```python
from build123d import *

# Parameters (mm, degrees)
F0_W     = 17.78
F0_H     = 73.152
F0_H_2   = 5.08
F1_DEPTH = 5.08
F2_DEPTH = 10.16
F4_DEPTH = 25.4


# Not quite as in the source:
# - a feature names something its author has since deleted; it is built from what else it names


with BuildPart() as f1:
    # F0 (on Top) → F1 (new body)
    with BuildSketch(Plane.XY):
        with Locations((8.89, -41.656)):
            Rectangle(F0_W, F0_H)
        with Locations((8.89, -2.54)):
            Rectangle(F0_W, F0_H_2)
        with Locations((8.89, -114.808)):
            Rectangle(F0_W, F0_H)
        with Locations((8.89, -153.924)):
            Rectangle(F0_W, F0_H_2)
    extrude(amount=-F1_DEPTH)

    # F0 (on Top) → F2 (join)
    with BuildSketch(Plane.XY):
        with Locations((8.89, -2.54)):
            Rectangle(F0_W, F0_H_2)
        with Locations((8.89, -153.924)):
            Rectangle(F0_W, F0_H_2)
    extrude(amount=F2_DEPTH)

    # F3 (on face) → F4 (cut)
    with BuildSketch(Plane(origin=(0, 0, 0), x_dir=(0, -1, 0), z_dir=(-1, 0, 0))):
        Polygon((3.048, 9.144), (5.08, 2.54), (5.08, 9.144), align=None)
        Polygon((151.384, 9.144), (151.384, 2.54), (153.416, 9.144), align=None)
    extrude(amount=-F4_DEPTH, mode=Mode.SUBTRACT)


solid = f1.part
```
Geometry check sheet. Reference: the model listing, model coordinates, mm. A direction names the side the tool comes from. Coordinates: 2 decimals unless noted, no trailing zeros. Loops run counter-clockwise (first coordinate to the right, second up) from the corner with the lowest first, then second, coordinate; pieces in that order, holes last. Notation, with made-up numbers: (-27.75, 12.25) -> (28.25, 12.25) arc R14 ccw to (28.25, 19.25) -> close; hole circle Ø4 at (-36.75, 89.25). An arc over 180 degrees is marked (long way). Put each result on its own line as item: value.
1) Cross-section at C-C on y = -121.5. Record the boundary of the cut face in (x, z).
Result set:
outline: (0, -5.08) -> (17.78, -5.08) -> (17.78, 0) -> (0, 0) -> close
2) Release check for a two-part mould opening along Z. For faces 4 (the flat face through (8.77, -4.05, 5.89)), 5 (the flat face through (9, -154, 10.16)), 6 (the flat face through (9, -5.08, 1)) record: released by +Z, released by -Z, zero draft, split by the parting line, or undercut.
Result set:
face 4: undercut
face 5: released by +Z
face 6: zero draft
3) Thickness scan on line 1 (Y direction, x = 4, z = 9.5); line 2 (Z direction, x = 7, y = -149); line 3 (Y direction, x = 14, z = 3). Record the ranges inside material, lowest first.
Result set:
line 1: y = -156.46 to -151.38, -5.08 to 0
line 2: z = -5.08 to 0
line 3: y = -156.46 to -151.53, -4.94 to 0
4) Gauge pin test, flat end, axial feed: pin 1 Ø10 at (x, y) = (13.5, -37.5) entering from +Z. Record the tip position at first contact, or that the pin passes through.
Result set:
pin 1: stops at z = 0
5) Cross-section at A-A on z = 6. Record the boundary of the cut face in (x, y).
Result set:
outline: (0, -156.46) -> (17.78, -156.46) -> (17.78, -152.45) -> (0, -152.45) -> close; (0, -4.02) -> (17.78, -4.02) -> (17.78, 0) -> (0, 0) -> close
6) Tool access check on faces 1 (the flat face through (9, -77, -5.08)), 2 (the flat face through (9, -77, 0)), 3 (the flat face through (8.766, -152.386, 5.796)). Record the directions out of +Z, -Z, +X, -X, +Y, -Y that give a thin tool (end or side, any length) a straight path to the whole face; none if there is none.
Result set:
face 1: -Z, +X, -X, +Y, -Y
face 2: +Z, +X, -X
face 3: +X, -X
7) Cross-section at B-B on x = 8.5. Record the boundary of the cut face in (y, z), plus the area to 3 significant figures.
Result set:
outline: (-156.46, -5.08) -> (0, -5.08) -> (0, 10.16) -> (-5.08, 10.16) -> (-5.08, 9.14) -> (-3.05, 9.14) -> (-5.08, 2.54) -> (-5.08, 0) -> (-151.38, 0) -> (-151.38, 2.54) -> (-153.42, 9.14) -> (-151.38, 9.14) -> (-151.38, 10.16) -> (-156.46, 10.16) -> close
area: 885 mm^2
